Could you check a few things on this model? Use its own coordinates, in mm. Give positions to 0.01 mm unless a question says otherwise; leave off trailing zeros. Loops run counter-clockwise (first coordinate to the right, second up) from the corner with the lowest first, then second, coordinate; pieces in that order, holes last. Notation, with made-up numbers: M 79,-11.75 L 133,-11.75 A24 cw 133,5.25 Z; hole C -11,-7 d6. An arc over 180 degrees is marked long. Write each question's results on one line, items separated by ' | '. Start each with the question number.
from build123d import *

# Parameters (mm, degrees)
SKETCH2_OUTSIDE_W  = 43.152
SKETCH2_OUTSIDE_H  = 43.152
CUT_EXTRUDE2_DEPTH = 25.4


with BuildPart() as part:
    # Sketch1 → Revolve1 (revolve)
    with BuildSketch(Plane(origin=(0, 0, 0), x_dir=(0, 0, -1), z_dir=(1, 0, 0)), mode=Mode.PRIVATE) as revolve1_sk:
        Polygon((-1.584325, 6.746875), (-12.334875, 6.746875), (-13.9192, 8.3312), (-13.9192, 11.1125), (-11.169569343, 15.875), (-2.749630657, 15.875), (0, 11.1125), (0, 8.3312), align=None)
    revolve(revolve1_sk.sketch.rotate(Axis((0, 0, -10.380814409), (0, 0, 1)), 90), axis=Axis((0, 0, -10.380814409), (0, 0, 1)))

    # Sketch2 outside → Cut-Extrude2 (cut)
    with BuildSketch(Plane.XY):
        Rectangle(SKETCH2_OUTSIDE_W, SKETCH2_OUTSIDE_H)
        Polygon((0, 13.755485633), (-11.9126, 6.877742817), (-11.9126, -6.877742817), (0, -13.755485633), (11.9126, -6.877742817), (11.9126, 6.877742817), align=None, mode=Mode.SUBTRACT)
    extrude(amount=CUT_EXTRUDE2_DEPTH, mode=Mode.SUBTRACT)


solid = part.part
1) I'm going to push flat-ended pins straight in: P1, Ø5, axis at x = 4, z = 6, coming from the -Y side; P2, Ø4, axis at x = -4.5, y = -0.5, coming from the +Z side; P3, Ø1, axis at x = 6.5, y = -10.5, coming from the -Z side; P4, Ø1, axis at x = 7, z = 10, coming from the -Y side. Where does each tip first touch, or does it pass through?
2) If we section it at A-A on z = 11.75: Write out the boundary of the cut face in (x, y), plus the area to 3 significant figures.
3) If we section it at B-B on y = 0: Write out the boundary of the cut face in (x, z).
4) Thinking about a two-plate mould opening in X: for faces 1 (the face through (-4.2, 7.4, 13.919)), 2 (the face through (-5.873, 10.365, 6.869)), 3 (the face through (4.97, -4.56, 7.03)), which applies, pulls with the +X half, pulls with the -X half, needs draft (parallel to the pull), parting line crosses it, or undercut?
5) Please list where these lines run through material, in increasing order: line 1 (Y direction, x = 4.5, z = 11.5); line 2 (X direction, y = 4.75, z = 4.25); line 3 (X direction, y = 5.5, z = 10.75). Write a range as from..to.
Calculated:
1) P1: stops at y = -12.89 | P2: passes through | P3: stops at z = 0.43 | P4: stops at y = -10
2) outline: M -11.91,-6.88 L 0,-13.76 L 11.91,-6.88 L 11.91,6.88 L 0,13.76 L -11.91,6.88 Z; hole C 0,0 d13.49 | area: 349 mm2
3) outline: M -11.91,0.46 L -11.11,0 L -8.33,0 L -6.75,1.58 L -6.75,12.33 L -8.33,13.92 L -11.11,13.92 L -11.91,13.46 Z; M 6.75,1.58 L 8.33,0 L 11.11,0 L 11.91,0.46 L 11.91,13.46 L 11.11,13.92 L 8.33,13.92 L 6.75,12.33 Z
4) face 1: needs draft | face 2: pulls with the -X half | face 3: undercut
5) line 1: y = -11.16..-5.03, 5.03..11.16 | line 2: x = -11.91..-4.79, 4.79..11.91 | line 3: x = -11.91..-3.91, 3.91..11.91
